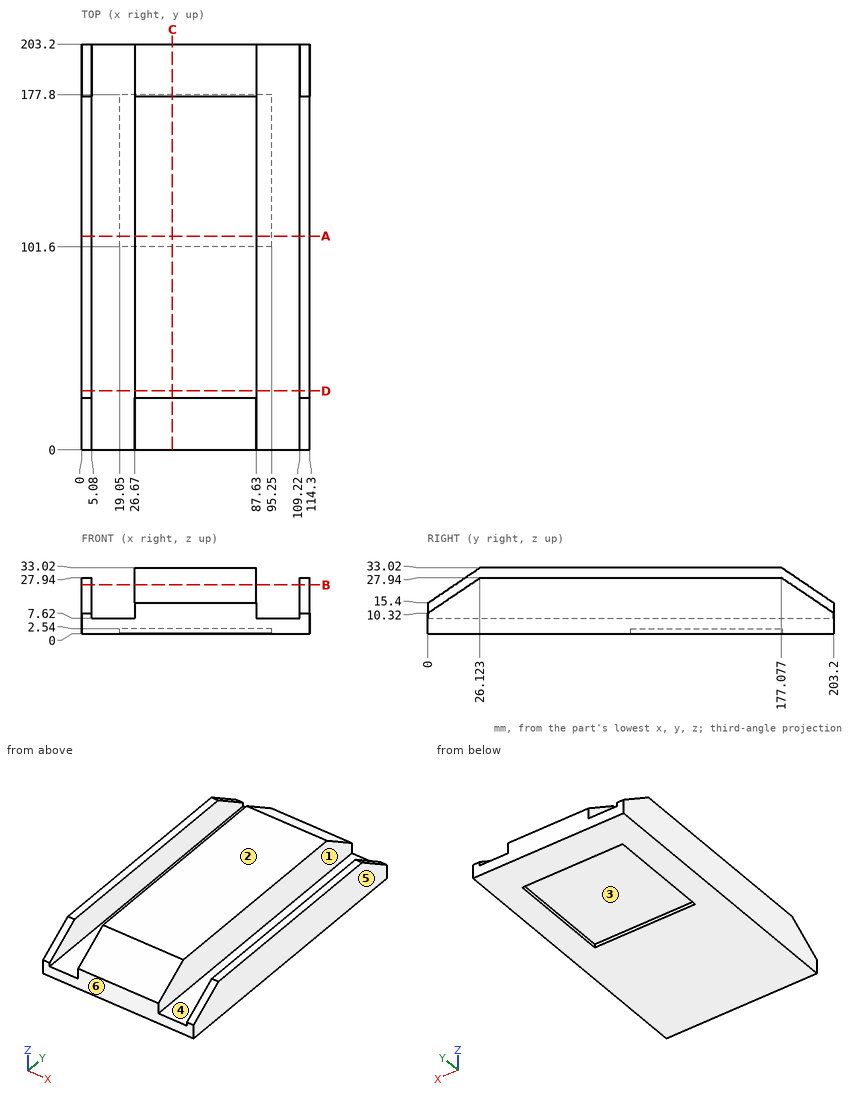
For this review, use the dimensioned drawing (mm, ordinates from the lowest corner) and the shaded views. A direction names the side the tool comes from. Round coordinates to 2 decimals unless told otherwise and drop trailing zeros. Write each loop counter-clockwise with the first axis right and the second up, starting at its lowest first coordinate (ties: lowest second). Pieces come first, ordered by that corner, then holes. Notation, with made-up numbers: (83.5, -16.75) -> (106.5, -16.75) arc R35 cw to (106.5, 16.25) -> close; hole circle Ø9 at (57.25, 58.5). An arc over 180 degrees is marked (long way). Use CSV: the item, a comma, the result in double quotes.
(1) Consider section A-A, the plane y = 107. Give the boundary of the cut face in (x, z).
Computed values:
outline,"(0, 0) -> (19.05, 0) -> (19.05, 2.54) -> (95.25, 2.54) -> (95.25, 0) -> (114.3, 0) -> (114.3, 27.94) -> (109.22, 27.94) -> (109.22, 7.62) -> (87.63, 7.62) -> (87.63, 33.02) -> (26.67, 33.02) -> (26.67, 7.62) -> (5.08, 7.62) -> (5.08, 27.94) -> (0, 27.94) -> close"
(2) Consider section D-D, the plane y = 29.5. Give the boundary of the cut face in (x, z).
Computed values:
outline,"(0, 0) -> (114.3, 0) -> (114.3, 27.94) -> (109.22, 27.94) -> (109.22, 7.62) -> (87.63, 7.62) -> (87.63, 33.02) -> (26.67, 33.02) -> (26.67, 7.62) -> (5.08, 7.62) -> (5.08, 27.94) -> (0, 27.94) -> close"
(3) Consider section B-B, the plane z = 24.5. Give the boundary of the cut face in (x, y).
Computed values:
outline,"(0, 21.02) -> (5.08, 21.02) -> (5.08, 182.18) -> (0, 182.18) -> close; (26.67, 13.49) -> (87.63, 13.49) -> (87.63, 189.71) -> (26.67, 189.71) -> close; (109.22, 21.02) -> (114.3, 21.02) -> (114.3, 182.18) -> (109.22, 182.18) -> close"
(4) To check wall thickness, follow L1, parallel to X at y = 43.5, z = 16; L2, parallel to Z at x = 89, y = 182; L3, parallel to Z at x = 89.5, y = 126. State the ranges of each line that lie inside material, in increasing order. Write a range as [from, to].
Computed values:
L1,"[0, 5.08], [26.67, 87.63], [109.22, 114.3]"
L2,"[0, 7.62]"
L3,"[2.54, 7.62]"
(5) For the marked faces 1, 2 and 3, list the 3-axis set-ups (+Z, -Z, +X, -X, +Y, -Y) from which the entire face can be reached by the end or side of a thin tool; tool diameter is ignored.
Computed values:
face 1,"+Z, +Y, -Y"
face 2,"+Z, +X, -X, +Y, -Y"
face 3,"-Z"
(6) Consider section C-C, the plane x = 45.5. Give the boundary of the cut face in (y, z).
Computed values:
outline,"(0, 0) -> (101.6, 0) -> (101.6, 2.54) -> (177.8, 2.54) -> (177.8, 0) -> (203.2, 0) -> (203.2, 15.4) -> (177.08, 33.02) -> (26.12, 33.02) -> (0, 15.4) -> close"
(7) Clearance check with flat-ended pins moving along their axes: P1, Ø23, axis at x = 51.5, y = 147.5, coming from the -Z side; P2, Ø6.5, axis at x = 10.5, y = 132, coming from the +Z side; P3, Ø4, axis at x = 1.5, y = 116, coming from the +Z side; P4, Ø1, axis at x = 34, y = 80.5, coming from the -Z side. State where each tip first meets the part, or that it passes through.
Computed values:
P1,"z = 2.54"
P2,"z = 7.62"
P3,"z = 27.94"
P4,"z = 0"
(8) Draft analysis for pull direction X (two halves, no side actions). For the marked faces 4, 5 and 6, state which applies: +X half, -X half, draft (parallel to the pull), parting line (faces both ways), or undercut.
Computed values:
face 4,"undercut"
face 5,"+X half"
face 6,"draft"
